Check sheet for the modelled part. Datum: model origin and axes. Units: mm. Face numbers are marked on the shaded views. Give positions to 0.01 mm unless a question says otherwise; leave off trailing zeros. Write each loop counter-clockwise with the first axis right and the second up, starting at its lowest first coordinate (ties: lowest second). Pieces come first, ordered by that corner, then holes. Notation, with made-up numbers: M 35,-37.75 L 93,-37.75 A15 cw 93,-30.75 Z; hole C -28,40.25 d6. An arc over 180 degrees is marked long. Write each question's results on one line, items separated by ' | '. Start each with the question number.
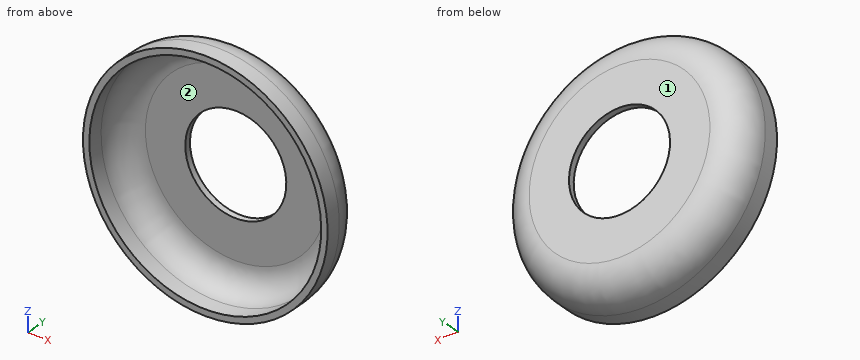
from build123d import *

# Parameters (mm, degrees)
SKETCH1_R           = 11.5
BOSS_EXTRUDE1_DEPTH = 4.5
FILLET2_R           = 3
SHELL1_T            = -0.6
SKETCH2_R           = 4.75
CUT_EXTRUDE1_DEPTH  = 17.874537031


with BuildPart() as part:
    # Sketch1 → Boss-Extrude1 (new body)
    with BuildSketch(Plane(origin=(0, 0, 0), x_dir=(1, 0, 0), z_dir=(0, 1, 0))):
        with Locations(Location((0, 0, 0), (0, 0, 270))):
            Circle(SKETCH1_R)
    extrude(amount=BOSS_EXTRUDE1_DEPTH)

    # Fillet2
    fillet2_edges = [part.edges().sort_by_distance(p)[0] for p in [
        (0, 4.5, -11.5),
    ]]
    fillet(fillet2_edges, radius=FILLET2_R)

    # Shell1
    shell1_openings = [part.faces().sort_by_distance(p)[0] for p in [
        (0, 0, 0),
    ]]
    offset(amount=SHELL1_T, openings=shell1_openings, kind=Kind.INTERSECTION)

    # Sketch2 → Cut-Extrude1 (cut, through all)
    with BuildSketch(Plane(origin=(0, 4.5, 0), x_dir=(1, 0, 0), z_dir=(0, 1, 0))):
        with Locations(Location((0, 0, 0), (0, 0, 270))):
            Circle(SKETCH2_R)
    extrude(amount=-CUT_EXTRUDE1_DEPTH, mode=Mode.SUBTRACT)


solid = part.part
Q1. Section check D-D on y = 3.6. Record the boundary of the cut face in (x, z), plus the area to 3 significant figures.
Q2. Depth check by flat-ended pin: pin 1 Ø1 at (x, z) = (-1.5, -2) entering from +Y; pin 2 Ø2 at (x, y) = (3.5, 2.5) entering from -Z; pin 3 Ø13 at (x, z) = (0, 0) entering from -Y; pin 4 Ø10 at (x, z) = (-1, -8.5) entering from -Y. Enter the tip coordinate at first touch or a pass-through.
Q3. Section check B-B on x = 0. Record the boundary of the cut face in (y, z), plus the area to 3 significant figures.
Q4. Section check C-C on y = 1.15. Record the boundary of the cut face in (x, z), plus the area to 3 significant figures.
Q5. Scan lines: L1, parallel to X at y = 0.6, z = 0; L2, parallel to Y at x = -1.5, z = -7.5; L3, parallel to X at y = 2.95, z = 1.25. Record each from-to range of solid material in increasing order.
Q6. Release check for a two-part mould opening along Z. For the marked faces 1 and 2 record: pulls with the +Z half, pulls with the -Z half, needs draft (parallel to the pull), parting line crosses it, or undercut.
Q7. Section check A-A on z = 0. Record the boundary of the cut face in (x, y).
Check result:
1) outline: C 0,0 d21.28; hole C 0,0 d19.32 | area: 62.5 mm^2
2) pin 1: through | pin 2: z = -11.15 | pin 3: y = 3.9 | pin 4: y = 0
3) outline: M 0,-11.5 L 1.5,-11.5 A3 ccw 4.5,-8.5 L 4.5,-4.75 L 3.9,-4.75 L 3.9,-8.5 A2.4 cw 1.5,-10.9 L 0,-10.9 Z; M 0,10.9 L 1.5,10.9 A2.4 cw 3.9,8.5 L 3.9,4.75 L 4.5,4.75 L 4.5,8.5 A3 ccw 1.5,11.5 L 0,11.5 Z | area: 11.4 mm^2
4) outline: C 0,0 d23; hole C 0,0 d21.8 | area: 42.2 mm^2
5) L1: -11.5 to -10.9, 10.9 to 11.5 | L2: 3.9 to 4.5 | L3: -11.06 to -10.34, 10.34 to 11.06
6) face 1: needs draft | face 2: undercut
7) outline: M -11.5,0 L -10.9,0 L -10.9,1.5 A2.4 cw -8.5,3.9 L -4.75,3.9 L -4.75,4.5 L -8.5,4.5 A3 ccw -11.5,1.5 Z; M 4.75,3.9 L 8.5,3.9 A2.4 cw 10.9,1.5 L 10.9,0 L 11.5,0 L 11.5,1.5 A3 ccw 8.5,4.5 L 4.75,4.5 Z
